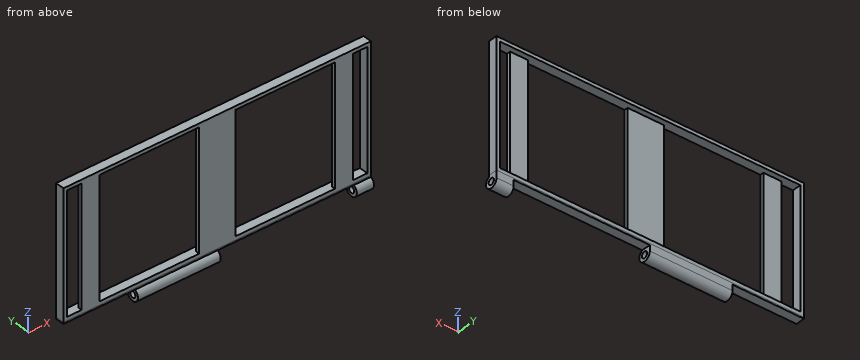
Autodesk Inventor part; units mm, degrees
ref_plane "YZ Plane" through (0, 0, 0) normal (1, 0, 0) x (0, 1, 0)
ref_plane "XZ Plane" through (0, 0, 0) normal (0, 1, 0) x (-1, 0, 0)
ref_plane "XY Plane" through (0, 0, 0) normal (0, 0, 1) x (1, 0, 0)
sketch "Skizze1" plane through (0, 0, 0) normal (0, 1, 0) x (-1, 0, 0)
  line L0 (0, 0) -> (-170, 0)
  line L1 (-170, 0) -> (-170, -70)
  line L2 (-170, -70) -> (0, -70)
  line L3 (0, -70) -> (0, 0)
  dimension "d0" = 170
  dimension "d1" = 70
extrude "Extrusion1" add sketch "Skizze1" along normal blind 5
sketch "Skizze2" plane through (0, 5, 0) normal (0, 1, 0) x (1, 0, 0)
  line L0 (170, 0) -> (170, 70)
  line L1 (170, 70) -> (0, 70)
  line L2 (0, 70) -> (0, 0)
  line L3 (0, 0) -> (170, 0)
  line L4 (2, 68) -> (168, 68)
  line L5 (168, 68) -> (168, 2)
  line L6 (168, 2) -> (2, 2)
  line L7 (2, 2) -> (2, 68)
  dimension "d4" = 2
extrude "Extrusion2" cut sketch "Skizze2" against normal blind 3 contours L4 L5 L6 L7
sketch "Skizze3" plane through (0, 2, 0) normal (0, 1, 0) x (1, 0, 0)
  line L0 (168, 2) -> (2, 2)
  line L1 (168, 68) -> (168, 2)
  line L2 (2, 68) -> (168, 68)
  line L3 (2, 2) -> (2, 68)
  line L4 (75, 68) -> (95, 68)
  line L5 (95, 68) -> (95, 2)
  line L6 (95, 2) -> (75, 2)
  line L7 (75, 2) -> (75, 68)
  line L8 (2, 68) -> (168, 68)
  line L9 (2, 68) -> (168, 68)
  line L10 (10, 68) -> (20, 68)
  line L11 (20, 68) -> (20, 2)
  line L12 (20, 2) -> (10, 2)
  line L13 (10, 2) -> (10, 68)
  line L14 (168, 2) -> (2, 2)
  line L15 (160, 68) -> (150, 68)
  line L16 (150, 68) -> (150, 2)
  line L17 (150, 2) -> (160, 2)
  line L18 (160, 2) -> (160, 68)
  line L19 (0, 70) -> (0, 0)
  line L20 (170, 0) -> (170, 70)
  point P0 (85, 68)
  point P1 (85, 68)
  point P2 (160, 2)
  point P3 (10, 2)
  dimension "d7" = 20
  dimension "d8" = 10
  dimension "d9" = 10
  dimension "d10" = 10
extrude "Extrusion3" cut sketch "Skizze3" against normal through all contours L0 L18 L2 L1 | L0 L5 L2 L16 | L0 L11 L2 L7 | L0 L3 L2 L13
sketch "Skizze4" plane through (170, 0, 0) normal (1, 0, 0) x (0, 0, -1)
  circle A0 centre (74, 1.5) radius 3.5
  circle A1 centre (74, 1.5) radius 1.75
  line L0 (0, 0) -> (70, 0)
  line L1 (0, 5) -> (70, 5)
  line L2 (70, 5) -> (74, 5)
  line L3 (70, 0) -> (70, 5)
  line L4 (70, 0) -> (70.8377, 0)
  point P0 (70, 3)
  dimension "d13" = 7
  dimension "d14" = 3.5
  dimension "d27" = 4
extrude "Extrusion4" add sketch "Skizze4" against normal up to surface (170 mm away)
sketch "Skizze5" plane through (0, 5, 0) normal (0, 1, 0) x (1, 0, 0)
  line L0 (170, 70.8377) -> (0, 70.8377)
  line L1 (170, 77.5) -> (0, 77.5)
  line L2 (170, 70.8377) -> (170, 77.5)
  line L3 (0, 70.8377) -> (0, 77.5)
  line L4 (170, 77.5) -> (0, 77.5)
  line L5 (9.5, 77.5) -> (9.5, 70.8377)
  line L6 (39.5, 70.8377) -> (39.5, 77.5)
  line L7 (160.5, 70.8377) -> (160.5, 77.5)
  line L8 (170, 77.5) -> (0, 77.5)
  line L9 (130.5, 70.8377) -> (130.5, 77.5)
  line L10 (85.25, 70.8377) -> (85.25, 77.5)
  line L11 (170, 77.5) -> (0, 77.5)
  line L12 (84.75, 77.5) -> (84.75, 70.8377)
  line L13 (85.25, 74.1094) -> (84.75, 74.1094) construction
  point P0 (0, 0)
  point P1 (85, 74.1094)
  point P2 (85, 77.5)
  dimension "d28" = 0.5
  dimension "d29" = 9.5
  dimension "d30" = 9.5
  dimension "d31" = 30
  dimension "d32" = 30
extrude "Extrusion5" cut sketch "Skizze5" against normal through all contours L0 L9 L1 L7 | L0 L10 L1 L9 | L0 L5 L1 L6 | L0 L3 L1 L5
equation "\"d9\" = d8"
equation "\"d30\" = d29"
equation "\"d32\" = d31"
properties part number "roof"
Geometry: final body of the model. Coordinates: model frame, mm. Give positions to 0.01 mm unless a question says otherwise; leave off trailing zeros. Order: outer loops, then holes, each group sorted by start corner. A loop starts at its lowest first (then second) coordinate and runs counter-clockwise, first axis right, second up. Notation, with made-up numbers: (26, 18) -> (82, 18) arc R21 cw to (82, 44) -> close; hole circle Ø4 at (22.5, 32). An arc over 180 degrees is marked (long way). Write each question's results on one line, items separated by ' | '. Start each with the question number.
1) Section C-C (x = 88). Return loops of the section in (y, z), then the cut area to 3 significant figures.
2) Section A-A (x = 33.5). Return loops of the section in (y, z).
3) First-contact query: pin 1 (5 mm diameter, centred on x = 15.5, z = -39, fed in from +Y); pin 2 (4 mm diameter, centred on x = 21, y = 1.5, fed in from -Z); pin 3 (3 mm diameter, centred on y = 1.5, z = -74, fed in from +X); pin 4 (4 mm diameter, centred on y = 1.5, z = -74, fed in from -X). Flat tips, straight axial feed; report the tip coordinate or a pass-through.
4) Line query: line 1 (X direction, y = 1.5, z = -65); line 2 (Y direction, x = 76, z = -74); line 3 (Z direction, x = 114.5, y = 2.75). Output: solid intervals per line, ascending. Write a range as from..to.
5) Section B-B (z = -49.5). Return loops of the section in (x, y), then the cut area to 3 significant figures.
Calculated:
1) outline: (0, -70.84) -> (5, -70.84) -> (5, -68) -> (2, -68) -> (2, -2) -> (5, -2) -> (5, 0) -> (0, 0) -> close | area: 156 mm2
2) outline: (0, -70.84) -> (5, -70.84) -> (5, -68) -> (0, -68) -> close; (0, -2) -> (5, -2) -> (5, 0) -> (0, 0) -> close
3) pin 1: y = 2 | pin 2: z = -70.84 | pin 3: through | pin 4: x = 39.5
4) line 1: 0..2, 10..20, 75..95, 150..160, 168..170 | line 2: -2..-0.25, 3.25..5 | line 3: -70.84..-68, -2..0
5) outline: (0, 0) -> (2, 0) -> (2, 5) -> (0, 5) -> close; (10, 0) -> (20, 0) -> (20, 2) -> (10, 2) -> close; (75, 0) -> (95, 0) -> (95, 2) -> (75, 2) -> close; (150, 0) -> (160, 0) -> (160, 2) -> (150, 2) -> close; (168, 0) -> (170, 0) -> (170, 5) -> (168, 5) -> close | area: 100 mm2
